```python
from build123d import *

# Parameters (mm, degrees)
F0_W     = 101.6
F0_H     = 7.493
F1_DEPTH = 63.5
F3_W     = 11.43
F3_H     = 7.493
F4_DEPTH = 24.13


with BuildPart() as f1:
    # F0 (on Right) → F1 (new body)
    with BuildSketch(Plane.YZ):
        with Locations((-50.8, 3.7465)):
            Rectangle(F0_W, F0_H)
    extrude(amount=F1_DEPTH)

    # F3 (on face) → F4 (join)
    with BuildSketch(Plane.XZ.offset(101.6)):
        with Locations((31.613354, 3.7465)):
            Rectangle(F3_W, F3_H)
    extrude(amount=F4_DEPTH)


solid = f1.part
```
Source: CAD feature listing. Evaluate the final solid. Frame: model axes, mm. A direction names the side the tool comes from. Give positions to 0.01 mm unless a question says otherwise; leave off trailing zeros. Order: outer loops, then holes, each group sorted by start corner. A loop starts at its lowest first (then second) coordinate and runs counter-clockwise, first axis right, second up.
(1) Access query for faces 1 (the face through (25.898, -113, 4)), 2 (the face through (37.328, -113, 4)), 3 (the face through (63.5, -52, 4)). Directions: +Z, -Z, +X, -X, +Y, -Y. A direction counts if a zero-diameter tool reaches every point of the face in a straight line with its end or side. Return the directions, or none.
(2) Contact query for flat-ended pins moving along their axis: P1, Ø3.5, axis at y = -114, z = 4.5, coming from the -X side; P2, Ø2, axis at x = 19, z = 1, coming from the -Y side; P3, Ø3.5, axis at y = -109.5, z = 3.5, coming from the +X side; P4, Ø6, axis at x = 8.5, y = -55.5, coming from the -Z side. Output: stop coordinate, or through.
(3) Section query B-B (x = 55). Return the cut outline in (y, z), plus the area to 3 significant figures.
(4) Section query A-A (z = 6). Return the cut outline in (x, y).
(5) Material intervals for line 1 along Y through (x, z) = (6.5, 1); line 2 along X through (y, z) = (-104, 3.25), sorted ascending.
Outcome:
1. face 1: +Z, -Z, -X, -Y
1. face 2: +Z, -Z, +X, -Y
1. face 3: +Z, -Z, +X, +Y, -Y
2. P1: stops at x = 25.9
2. P2: stops at y = -101.6
2. P3: stops at x = 37.33
2. P4: stops at z = 0
3. outline: (-101.6, 0) - (0, 0) - (0, 7.49) - (-101.6, 7.49) - close
3. area: 761 mm2
4. outline: (0, -101.6) - (25.9, -101.6) - (25.9, -125.73) - (37.33, -125.73) - (37.33, -101.6) - (63.5, -101.6) - (63.5, 0) - (0, 0) - close
5. line 1: y = -101.6 to 0
5. line 2: x = 25.9 to 37.33
